Autodesk Inventor part; units mm, degrees
ref_plane "XZ Plane" through (0, 0, 0) normal (0, 1, 0) x (-1, 0, 0)
sketch "Sketch5" plane through (0, 0, 0) normal (0, 1, 0) x (-1, 0, 0)
  line L0 (0, 0) -> (0, 247.65) construction
  line L1 (0, 0) -> (304.8, 0) construction
  line L2 (0, 247.65) -> (304.8, 247.65)
  line L3 (304.8, 247.65) -> (304.8, 0)
  dimension "d11" = 247.65
  dimension "d12" = 304.8
sketch "Sketch6" plane through (0, 0, 0) normal (1, 0, 0) x (0, 1, 0)
  line L0 (-12.7, 260.35) -> (-12.7, 234.95)
  line L1 (-12.7, 234.95) -> (12.7, 234.95)
  line L2 (12.7, 234.95) -> (12.7, 260.35)
  line L3 (12.7, 260.35) -> (-12.7, 260.35)
  line L4 (-12.7, 260.35) -> (12.7, 234.95) construction
  line L5 (-12.7, 234.95) -> (12.7, 260.35) construction
  point P0 (0, 0)
  point P1 (0, 247.65)
  dimension "d13" = 25.4
  dimension "d14" = 25.4
  dimension "d15" = 247.65
sweep "Sweep2" add profiles "Sketch6" path "Sketch5"
ref_plane "Work Plane1" through (-304.8, 0, 0) normal (1, 0, 0) x (0, 1, 0)
equation "\"d11\" = width"
equation "\"d12\" = length"
equation "\"width\" = 247.65"
equation "\"length\" = 304.8"
equation "\"d18\" = -length"
equation "\"height\" = 241.3"
properties part number "topOfFrame"
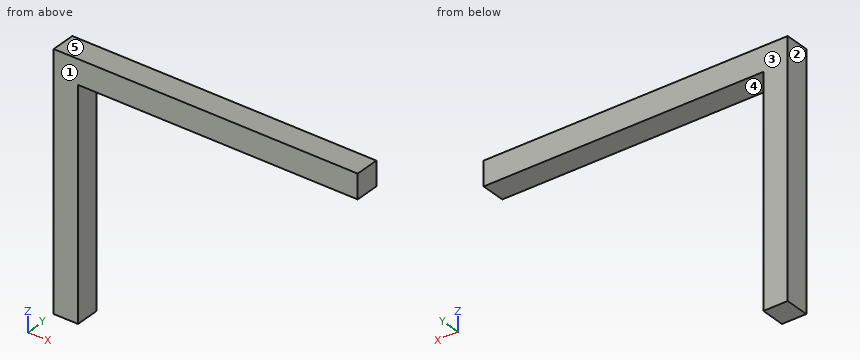
CAD build for the part. Positions are in the model's coordinates, mm. Face numbers are marked on the shaded views. A direction names the side the tool comes from. Coordinates: 2 decimals unless noted, no trailing zeros. Order: outer loops, then holes, each group sorted by start corner. A loop starts at its lowest first (then second) coordinate and runs counter-clockwise, first axis right, second up.
(1) Saw through at C-C, the plane x = -195. Write the cut outline in (y, z).
Solution:
outline: (-12.7, 234.95) - (12.7, 234.95) - (12.7, 260.35) - (-12.7, 260.35) - close
(2) Saw through at A-A, the plane y = -8.75. Write the cut outline in (x, z).
Solution:
outline: (-317.5, 0) - (-292.1, 0) - (-292.1, 234.95) - (0, 234.95) - (0, 260.35) - (-317.5, 260.35) - close
(3) Which spindle directions (+Z, -Z, +X, -X, +Y, -Y) get a long thin tool onto all of the face, cutting with end or side? Do the marked faces 4 and 5. Say none if no direction does.
Solution:
face 4: -Z, +X, +Y, -Y
face 5: +Z, +X, -X, +Y, -Y
(4) Pin check, flat tips, straight feed: pin 1 Ø1 at (y, z) = (6.5, 41) entering from +X; pin 2 Ø3 at (x, y) = (-158.5, -1.5) entering from -Z. Stop position of each tip, or through.
Solution:
pin 1: stops at x = -292.1
pin 2: stops at z = 234.95
(5) Saw through at B-B, the plane z = 38. Write the cut outline in (x, y).
Solution:
outline: (-317.5, -12.7) - (-292.1, -12.7) - (-292.1, 12.7) - (-317.5, 12.7) - close
(6) Drill centre lines: L1, parallel to X at y = -5.5, z = 50; L2, parallel to Z at x = -107, y = -8.5. Where is each one in solid material? Low to high.
Solution:
L1: x = -317.5 to -292.1
L2: z = 234.95 to 260.35
(7) Mould opens along Y. For the marked faces 1, 2 and 3 say: released by +Y, released by -Y, zero draft, split by the parting line, or undercut.
Solution:
face 1: released by -Y
face 2: zero draft
face 3: released by +Y
